Geometry check sheet. Reference: the model listing, model coordinates, mm. A direction names the side the tool comes from. Give positions to 0.01 mm unless a question says otherwise; leave off trailing zeros. Write each loop counter-clockwise with the first axis right and the second up, starting at its lowest first coordinate (ties: lowest second). Pieces come first, ordered by that corner, then holes.
(1) Depth check by flat-ended pin: P1, Ø1.7, axis at x = 20, z = 5.5, coming from the +Y side; P2, Ø3, axis at x = 34, y = -9.5, coming from the +Z side. Enter the tip coordinate at first touch or a pass-through.
(2) Mould release check, pull along Z, two halves, no side actions. Record for faces 4 (the cylindrical face through (22.747, -18.073, 5.121)), 5 (the flat face through (36.5, -12.54, 1.23)), 6 (the flat face through (37, -10, 7)), 7 (the cylindrical face through (17.97, -4.29, 6.86)): +Z half, -Z half, draft (parallel to the pull), parting line (faces both ways), or undercut.
(3) Cross-section at C-C (x = 27.5). Record the boundary of the cut face in (y, z), and give its area (3 significant figures).
(4) Cross-section at A-A (x = 5). Record the boundary of the cut face in (y, z), and give its area (3 significant figures).
(5) Thickness scan on line 1 along X through (y, z) = (-11.5, 0.5); line 2 along X through (y, z) = (-6.25, 5.75); line 3 along Z through (x, y) = (20, -2.6). Record the ranges inside material, lowest first.
(6) Cross-section at D-D (z = 5). Count the separate pieces of the cut face and the enclosed holes in it, and give its area (3 significant figures).
(7) Cross-section at B-B (y = -10). Record the boundary of the cut face in (x, z) (3 decimals), and give its area (3 significant figures).
(8) Tool access check on faces 1 (the flat face through (21, -4.8, 2)), 2 (the flat face through (20, -20, 2)), 3 (the flat face through (33.6, -8.5, 2.5)). Record the directions out of +Z, -Z, +X, -X, +Y, -Y that give a thin tool (end or side, any length) a straight path to the whole face; none if there is none.
```python
from build123d import *

# Parameters (mm, degrees)
SKETCH_W         = 40
SKETCH_H         = 20
SKETCH_W_2       = 20
SKETCH_H_2       = 12.4
PAD_DEPTH        = 10
HOLE_D           = 3.5
HOLE_DEPTH       = 25
HOLE_CBORE_D     = 5.75
HOLE_CBORE_DEPTH = 3
POCKET_DEPTH     = 2.5
SKETCH003_R      = 2.75
POCKET001_DEPTH  = 20.001
SKETCH004_R      = 3.5
SKETCH004_R_2    = 2.774564
PAD001_DEPTH     = 1
SKETCH005_R      = 3.5
SKETCH005_R_2    = 2.755211
PAD002_DEPTH     = 1
CHAMFER_SIZE     = 0.99


with BuildPart() as part:
    # Sketch → Pad (new body)
    with BuildSketch(Plane.XY):
        with Locations((20, -10)):
            Rectangle(SKETCH_W, SKETCH_H)
        with Locations((20, -10)):
            Rectangle(SKETCH_W_2, SKETCH_H_2, mode=Mode.SUBTRACT)
    extrude(amount=PAD_DEPTH)

    # Hole
    with Locations(Plane.XY.offset(10)):
        with Locations((35, -10)):
            CounterBoreHole(HOLE_D / 2, HOLE_CBORE_D / 2, HOLE_CBORE_DEPTH, depth=HOLE_DEPTH)

    # Sketch002 (on Face4 of Hole) → Pocket (cut)
    with BuildSketch(Plane(origin=(0, 0, 0), x_dir=(1, 0, 0), z_dir=(0, 0, -1))):
        Polygon((37.95, 11.703183), (35, 13.406367), (32.05, 11.703183), (32.05, 8.296817), (35, 6.593633), (37.95, 8.296817), align=None)
    extrude(amount=-POCKET_DEPTH, mode=Mode.SUBTRACT)

    # Sketch003 (on Face1 of Pocket) → Pocket001 (cut, through all)
    with BuildSketch(Plane(origin=(0, 0, 0), x_dir=(-1, 0, 0), z_dir=(0, 1, 0))):
        with Locations((-5, 5)):
            Circle(SKETCH003_R)
        with Locations((-20, 5)):
            Circle(SKETCH003_R)
    extrude(amount=-POCKET001_DEPTH, mode=Mode.SUBTRACT)

    # Sketch004 (on Face16 of Pocket001) → Pad001 (join)
    with BuildSketch(Plane(origin=(0, -16.2, 0), x_dir=(-1, 0, 0), z_dir=(0, 1, 0))):
        with Locations((-20, 5)):
            Circle(SKETCH004_R)
        with Locations((-20, 5)):
            Circle(SKETCH004_R_2, mode=Mode.SUBTRACT)
    extrude(amount=PAD001_DEPTH)

    # Sketch005 (on Face17 of Pad001) → Pad002 (join)
    with BuildSketch(Plane.XZ.offset(3.8)):
        with Locations((20, 5)):
            Circle(SKETCH005_R)
        with Locations((20, 5)):
            Circle(SKETCH005_R_2, mode=Mode.SUBTRACT)
    extrude(amount=PAD002_DEPTH)

    # Chamfer
    chamfer_edges = [part.edges().sort_by_distance(p)[0] for p in [
        (16.5, -3.8, 5),
        (23.5, -16.2, 5),
    ]]
    chamfer(chamfer_edges, length=CHAMFER_SIZE)


solid = part.part
```
Reply:
1. P1: passes through
1. P2: stops at z = 7
2. face 4: undercut
2. face 5: draft
2. face 6: +Z half
2. face 7: undercut
3. outline: (-20, 0) - (-16.2, 0) - (-16.2, 10) - (-20, 10) - close; (-3.8, 0) - (0, 0) - (0, 10) - (-3.8, 10) - close
3. area: 76.0 mm2
4. outline: (-20, 0) - (0, 0) - (0, 2.25) - (-20, 2.25) - close; (-20, 7.75) - (0, 7.75) - (0, 10) - (-20, 10) - close
4. area: 90.0 mm2
5. line 1: x = 0 to 10, 30 to 32.05, 37.95 to 40
5. line 2: x = 0 to 2.35, 7.65 to 10, 30 to 40
5. line 3: z = 0 to 2.25, 7.75 to 10
6. separate pieces: 3
6. enclosed holes: 1
6. area: 395 mm2
7. outline: (0, 0) - (10, 0) - (10, 10) - (0, 10) - close; (30, 0) - (32.05, 0) - (32.05, 2.5) - (33.25, 2.5) - (33.25, 7) - (32.125, 7) - (32.125, 10) - (30, 10) - close; (36.75, 2.5) - (37.95, 2.5) - (37.95, 0) - (40, 0) - (40, 10) - (37.875, 10) - (37.875, 7) - (36.75, 7) - close; hole circle Ø5.5 at (5, 5)
7. area: 128 mm2
8. face 1: +Z, -Z
8. face 2: +Z, -Z, +X, -X, -Y
8. face 3: -Z
